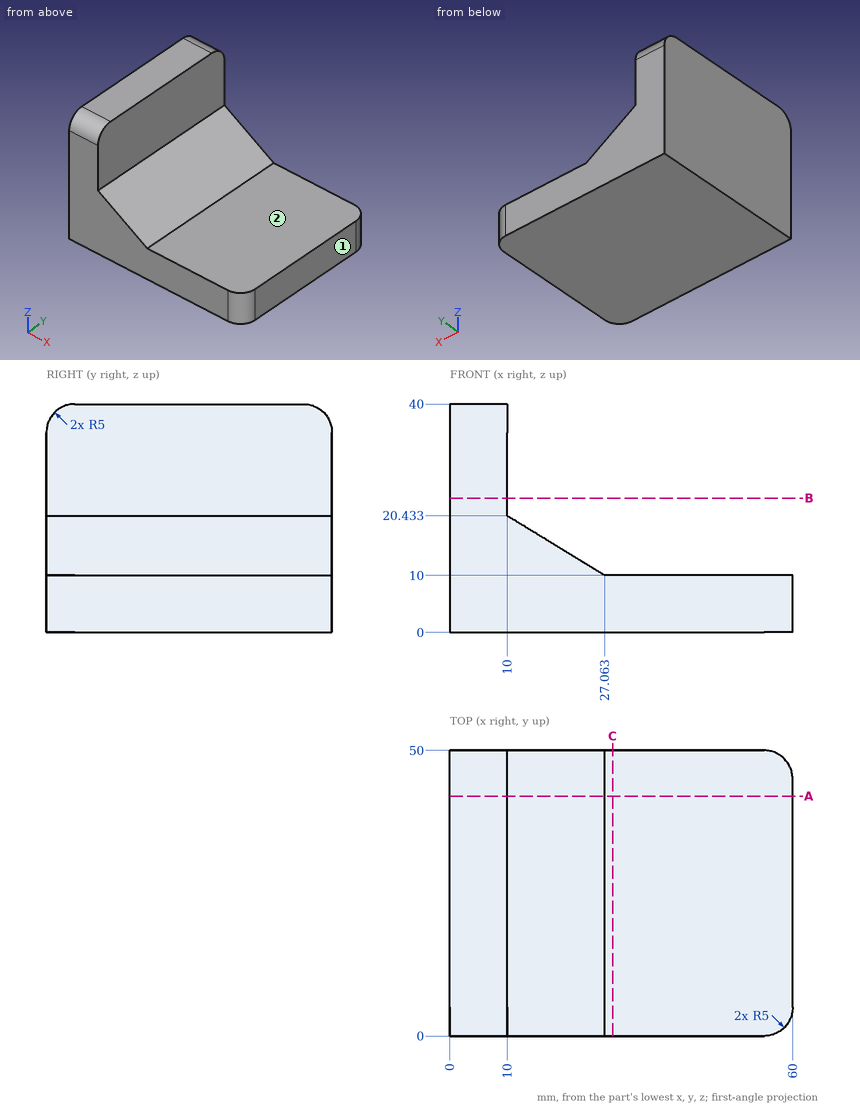
Source: three-view drawing plus pictorial views. Frame: mm from the lowest corner of the part. A direction names the side the tool comes from. Give positions to 0.01 mm unless a question says otherwise; leave off trailing zeros. Order: outer loops, then holes, each group sorted by start corner. A loop starts at its lowest first (then second) coordinate and runs counter-clockwise, first axis right, second up. Notation, with made-up numbers: M -23,88.5 L 24,88.5 A28 ccw 24,115.5 Z; hole C 52.25,-7 d9. An arc over 180 degrees is marked long. One line per question, with ' | ' between items. Start each with the question number.
1. Section query B-B (z = 23.5). Return the cut outline in (x, y), and give its area (3 significant figures).
2. Material intervals for probe 1 along X at (y, z) = (40.5, 22); probe 2 along Z at (x, y) = (11, 40.5), sorted ascending. Write a range as [from, to].
3. Section query A-A (y = 42). Return the cut outline in (x, z), and give its area (3 significant figures).
4. Section query C-C (x = 28.5). Return the cut outline in (y, z), and give its area (3 significant figures).
5. First-contact query: pin 1 Ø1 at (y, z) = (12, 7) entering from -X; pin 2 Ø6 at (y, z) = (16.5, 26.5) entering from +X; pin 3 Ø5 at (x, y) = (29, 14) entering from +Z (1 decimal); pin 4 Ø5 at (x, y) = (49.5, 29.5) entering from +Z. Flat tips, straight axial feed; report the tip coordinate or a pass-through.
6. Access query for the marked faces 1 and 2. Directions: +Z, -Z, +X, -X, +Y, -Y. A direction counts if a zero-diameter tool reaches every point of the face in a straight line with its end or side. Return the directions, or none.
Here are the results:
1) outline: M 0,0 L 10,0 L 10,50 L 0,50 Z | area: 500 mm²
2) probe 1: [0, 10] | probe 2: [0, 19.82]
3) outline: M 0,0 L 60,0 L 60,10 L 27.06,10 L 10,20.43 L 10,40 L 0,40 Z | area: 989 mm²
4) outline: M 0,0 L 50,0 L 50,10 L 0,10 Z | area: 500 mm²
5) pin 1: x = 0 | pin 2: x = 10 | pin 3: z = 10.3 | pin 4: z = 10
6) face 1: +Z, -Z, +X, +Y, -Y | face 2: +Z, +X, +Y, -Y
